from build123d import *

# Parameters (mm, degrees)
F1_DEPTH = 25.4
F2_R     = 6.354917
F3_DEPTH = 25.4
F5_DEPTH = 25.4


with BuildPart() as f1:
    # F0 (on Front) → F1 (new body)
    with BuildSketch(Plane.XZ):
        Polygon((0, 31.75), (0, 0), (69.85, 0), (69.85, 12.7), (25.4, 12.7), (25.4, 31.75), align=None)
    extrude(amount=F1_DEPTH)

    # F2 (on face) → F3 (cut)
    with BuildSketch(Plane.XZ.offset(25.4)):
        with BuildLine():
            ThreePointArc((12.7, 31.75), (21.680256, 28.030256), (25.4, 19.05))
            Line((25.4, 19.05), (25.4, 31.75))
            Line((25.4, 31.75), (12.7, 31.75))
        make_face()
        with BuildLine():
            ThreePointArc((0, 19.05), (3.719744, 28.030256), (12.7, 31.75))
            Line((12.7, 31.75), (0, 31.75))
            Line((0, 31.75), (0, 19.05))
        make_face()
        with Locations((12.7, 19.05)):
            Circle(F2_R)
    extrude(amount=-F3_DEPTH, mode=Mode.SUBTRACT)

    # F4 (on face) → F5 (cut)
    with BuildSketch(Plane.XY.offset(12.7)):
        with BuildLine():
            ThreePointArc((38.1, -19.05), (42.590128, -17.190128), (44.45, -12.7))
            ThreePointArc((44.45, -12.7), (42.590128, -8.209872), (38.1, -6.35))
            ThreePointArc((38.1, -6.35), (31.75, -12.7), (38.1, -19.05))
        make_face()
        with BuildLine():
            ThreePointArc((38.1, -6.35), (42.590128, -8.209872), (44.45, -12.7))
            ThreePointArc((44.45, -12.7), (42.590128, -17.190128), (38.1, -19.05))
            Line((38.1, -19.05), (57.15, -19.05))
            ThreePointArc((57.15, -19.05), (50.8, -12.7), (57.15, -6.35))
            Line((57.15, -6.35), (38.1, -6.35))
        make_face()
        with BuildLine():
            ThreePointArc((63.5, -12.7), (61.640128, -8.209872), (57.15, -6.35))
            ThreePointArc((57.15, -6.35), (50.8, -12.7), (57.15, -19.05))
            ThreePointArc((57.15, -19.05), (61.640128, -17.190128), (63.5, -12.7))
        make_face()
        with BuildLine():
            ThreePointArc((57.15, 0), (66.130256, -3.719744), (69.85, -12.7))
            Line((69.85, -12.7), (69.85, 0))
            Line((69.85, 0), (57.15, 0))
        make_face()
        with BuildLine():
            ThreePointArc((69.85, -12.7), (66.130256, -21.680256), (57.15, -25.4))
            Line((57.15, -25.4), (69.85, -25.4))
            Line((69.85, -25.4), (69.85, -12.7))
        make_face()
    extrude(amount=-F5_DEPTH, mode=Mode.SUBTRACT)


solid = f1.part
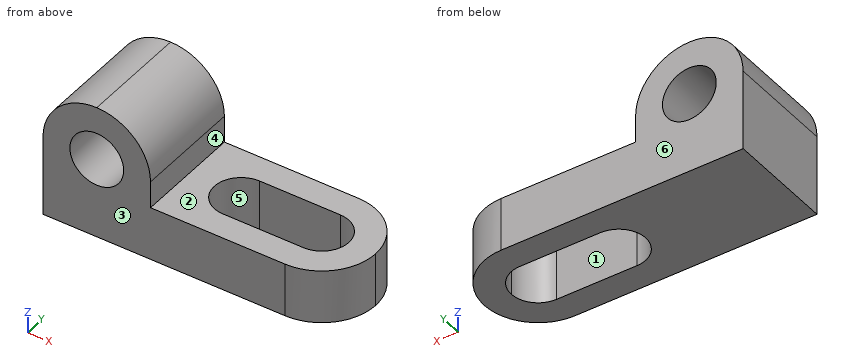
Build history of the part. All positions in model axes, mm. Face numbers are marked on the shaded views. A direction names the side the tool comes from. Round coordinates to 2 decimals unless told otherwise and drop trailing zeros. Loops run counter-clockwise (first coordinate to the right, second up) from the corner with the lowest first, then second, coordinate; pieces in that order, holes last. Notation, with made-up numbers: (86, -30.5) -> (120, -30.5) arc R17 cw to (120, -21.5) -> close; hole circle Ø7 at (64, 58). An arc over 180 degrees is marked (long way). Use CSV: the item, a comma, the result in double quotes. Start each with the question number.
Q1. Drill centre lines: L1, parallel to Z at x = 12.7, y = -6; L2, parallel to Y at x = 43.5, z = 10.5; L3, parallel to Z at x = 38, y = -2.5. Where is each one in solid material? Low to high.
Q2. Saw through at C-C on z = 11.5. Give the cut face in (x, y).
Q3. Saw through at D-D on z = 15.5. Give the cut face in (x, y), and give its area (3 significant figures).
Q4. Mould opens along Y. For the marked faces 4, 5 and 6 say: +Y half, -Y half, draft (parallel to the pull), parting line (faces both ways), or undercut.
Q5. Saw through at A-A on y = -8. Give the cut face in (x, z).
Q6. Saw through at B-B on x = 42. Give the cut face in (y, z), and give its area (3 significant figures).
Q7. Which spindle directions (+Z, -Z, +X, -X, +Y, -Y) get a long thin tool onto all of the face, cutting with end or side? Do the marked faces 1, 2 and 3. Say none if no direction does.
Q8. Flat gauge pins, fed straight in: pin 1 Ø1.5 at (x, y) = (57, -4.5) entering from +Z; pin 2 Ø1.5 at (y, z) = (-4.5, 6) entering from +X; pin 3 Ø2 at (y, z) = (-19.5, 6.5) entering from +X. Where does each tip first touch, or does it go through?
Solutions:
1,L1,"z = 0 to 12.7, 25.4 to 31.75"
1,L2,"y = -25.4 to -19.05, -6.35 to 0"
1,L3,"z = 0 to 12.7"
2,outline,"(0, -25.4) -> (57.15, -25.4) arc R12.7 ccw to (57.15, 0) -> (0, 0) -> close; hole (38.1, -19.05) -> (57.15, -19.05) arc R6.35 ccw to (57.15, -6.35) -> (38.1, -6.35) arc R6.35 ccw to start"
3,outline,"(0, -25.4) -> (7.43, -25.4) -> (7.43, 0) -> (0, 0) -> close; (17.97, -25.4) -> (25.4, -25.4) -> (25.4, 0) -> (17.97, 0) -> close"
3,area,"377 mm^2"
4,face 4,"draft"
4,face 5,"undercut"
4,face 6,"+Y half"
5,outline,"(0, 0) -> (33.83, 0) -> (33.83, 12.7) -> (25.4, 12.7) -> (25.4, 19.05) arc R12.7 ccw to (0, 19.05) -> close; (61.42, 0) -> (68.95, 0) -> (68.95, 12.7) -> (61.42, 12.7) -> close; hole circle Ø12.71 at (12.7, 19.05)"
6,outline,"(-25.4, 0) -> (-19.05, 0) -> (-19.05, 12.7) -> (-25.4, 12.7) -> close; (-6.35, 0) -> (0, 0) -> (0, 12.7) -> (-6.35, 12.7) -> close"
6,area,"161 mm^2"
7,face 1,"+Z, -Z"
7,face 2,"+Z, +X, +Y, -Y"
7,face 3,"+Z, -Z, +X, -X, -Y"
8,pin 1,"stops at z = 12.7"
8,pin 2,"stops at x = 67.44"
8,pin 3,"stops at x = 68.45"
